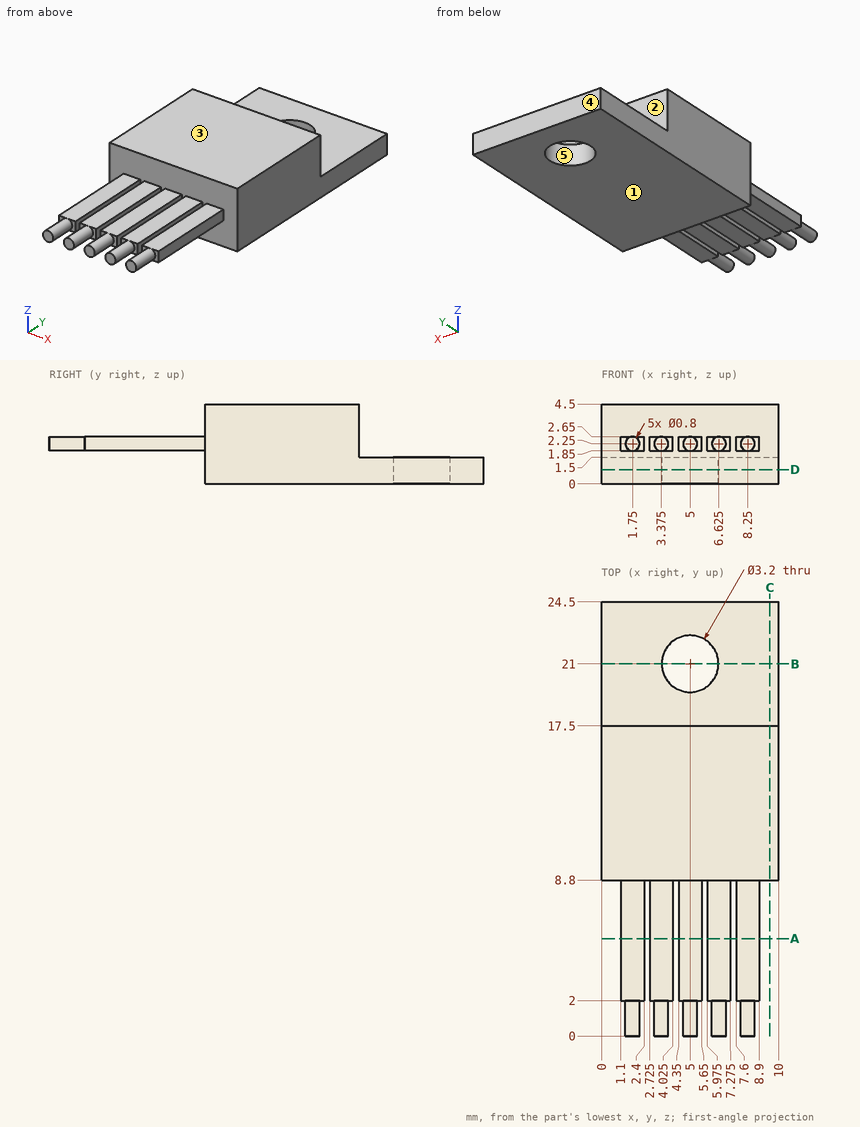
Study the drawing (mm; zero at the part's minimum x, y, z) and answer. A direction names the side the tool comes from. Round coordinates to 2 decimals unless told otherwise and drop trailing zeros. Loops run counter-clockwise (first coordinate to the right, second up) from the corner with the lowest first, then second, coordinate; pieces in that order, holes last.
Q1. Section B-B, the plane y = 21 is taken. Determine the outline of the cut face in (x, z).
Q2. Given pin 1 Ø1.4 at (x, y) = (1.5, 6) entering from -Z; pin 2 Ø0.6 at (y, z) = (4, 2) entering from -X; pin 3 Ø3.5 at (x, y) = (5, 19.5) entering from +Z; pin 4 Ø1 at (y, z) = (6.5, 1) entering from -X (3 decimals), each flat-ended and moving along its own axis, determine where each tip first touches the part or whether it passes through.
Q3. Find the intervals of material crossed by line 1 (X direction, y = 5, z = 2) (3 decimals); line 2 (Y direction, x = 5, z = 1); line 3 (Y direction, x = 4, z = 3.9), in increasing order.
Q4. Section D-D, the plane z = 0.8 is taken. Determine the outline of the cut face in (x, y).
Q5. Which of the six approach directions +Z, -Z, +X, -X, +Y, -Y give full straight-line access (tool end or side, diameter ignored) to the marked faces 1 and 2?
Q6. For a pull along Y with two mould halves and no side action, classify the marked faces 3, 4 and 5 as released by +Y, released by -Y, zero draft, split by the parting line, or undercut.
Q7. Section C-C, the plane x = 9.5 is taken. Determine the outline of the cut face in (y, z).
Q8. Section A-A, the plane y = 5.5 is taken. Determine the outline of the cut face in (x, z) (3 decimals).
Completed:
1. outline: (0, 0) - (3.4, 0) - (3.4, 1.5) - (0, 1.5) - close; (6.6, 0) - (10, 0) - (10, 1.5) - (6.6, 1.5) - close
2. pin 1: stops at z = 1.85
2. pin 2: stops at x = 1.1
2. pin 3: stops at z = 1.5
2. pin 4: passes through
3. line 1: x = 1.1 to 2.4, 2.725 to 4.025, 4.35 to 5.65, 5.975 to 7.275, 7.6 to 8.9
3. line 2: y = 8.8 to 19.4, 22.6 to 24.5
3. line 3: y = 8.8 to 17.5
4. outline: (0, 8.8) - (10, 8.8) - (10, 24.5) - (0, 24.5) - close; hole circle Ø3.2 at (5, 21)
5. face 1: -Z, +X, -X, +Y, -Y
5. face 2: +Z, +X, -X, +Y
6. face 3: zero draft
6. face 4: released by +Y
6. face 5: undercut
7. outline: (8.8, 0) - (24.5, 0) - (24.5, 1.5) - (17.5, 1.5) - (17.5, 4.5) - (8.8, 4.5) - close
8. outline: (1.1, 1.85) - (2.4, 1.85) - (2.4, 2.65) - (1.1, 2.65) - close; (2.725, 1.85) - (4.025, 1.85) - (4.025, 2.65) - (2.725, 2.65) - close; (4.35, 1.85) - (5.65, 1.85) - (5.65, 2.65) - (4.35, 2.65) - close; (5.975, 1.85) - (7.275, 1.85) - (7.275, 2.65) - (5.975, 2.65) - close; (7.6, 1.85) - (8.9, 1.85) - (8.9, 2.65) - (7.6, 2.65) - close
